Study the drawing (mm; zero at the part's minimum x, y, z) and answer. Give positions to 0.01 mm unless a question says otherwise; leave off trailing zeros. Write each loop counter-clockwise with the first axis right and the second up, starting at its lowest first coordinate (ties: lowest second). Pieces come first, ordered by that corner, then holes. Notation, with made-up numbers: (-35.75, 58) -> (17.25, 58) arc R27 cw to (17.25, 86) -> close; hole circle Ø1 at (74, 14). An arc over 180 degrees is marked (long way). Put each result on its own line as item: value. Start each with the question number.
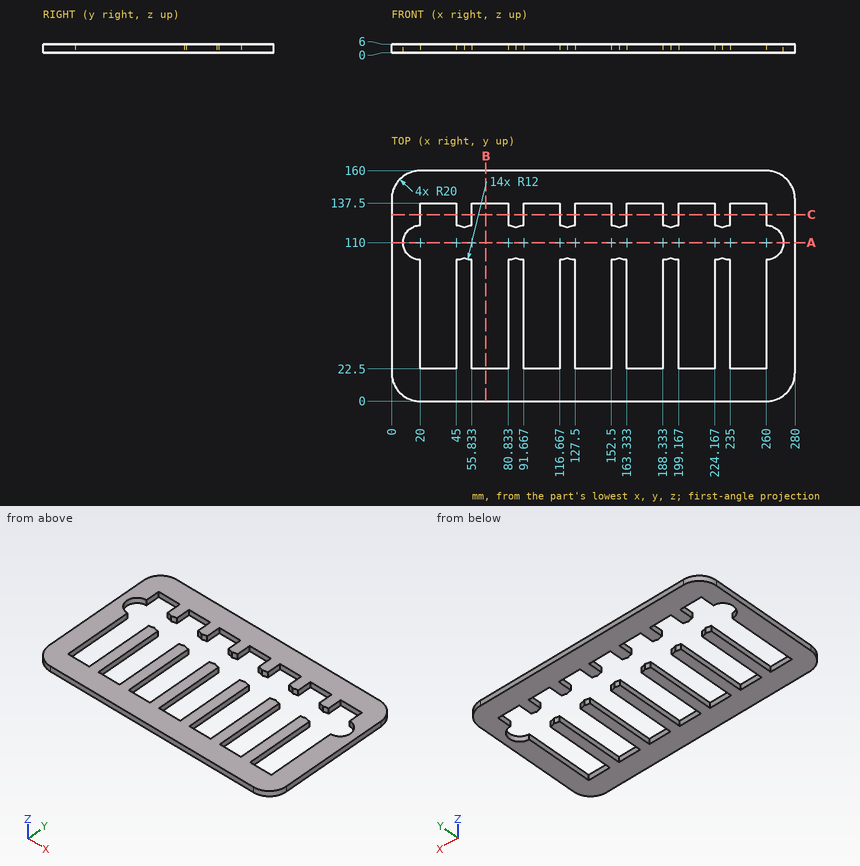
1) A cutting plane is placed at B-B on x = 65.5. Give the vertices of the cut face in (y, z), and give its area (3 significant figures).
2) A cutting plane is placed at C-C on y = 129.5. State how many separate pieces and enclosed holes the cut face has, and give its area (3 significant figures).
3) Straight lines are drawn through the part: line 1 (Y direction, x = 176, z = 3.1); line 2 (X direction, y = 111, z = 5.5); line 3 (Y direction, x = 15.5, z = 1.6) (1 decimal). For each, find the intervals that lie inside material, in ascending order. Write a range as [from, to].
4) A cutting plane is placed at A-A on y = 110. Give the vertices of the cut face in (x, z), and give its area (3 significant figures).
Results found:
1. outline: (0, 0) -> (22.5, 0) -> (22.5, 6) -> (0, 6) -> close; (137.5, 0) -> (160, 0) -> (160, 6) -> (137.5, 6) -> close
1. area: 270 mm²
2. separate pieces: 8
2. enclosed holes: 0
2. area: 630 mm²
3. line 1: y = [0, 22.5], [137.5, 160]
3. line 2: x = [0, 8.04], [271.96, 280]
3. line 3: y = [0.5, 98.9], [121.1, 159.5]
4. outline: (0, 0) -> (8, 0) -> (8, 6) -> (0, 6) -> close; (272, 0) -> (280, 0) -> (280, 6) -> (272, 6) -> close
4. area: 96.0 mm²
